Design review of the part built by this model. Coordinates are the model's own, in mm. A direction names the side the tool comes from. Round coordinates to 2 decimals unless told otherwise and drop trailing zeros. Order: outer loops, then holes, each group sorted by start corner. A loop starts at its lowest first (then second) coordinate and runs counter-clockwise, first axis right, second up. Notation, with made-up numbers: (58.5, 29.5) - (67.5, 29.5) arc R7 ccw to (67.5, 35.5) - close; hole circle Ø11 at (-36.75, 47.25). An arc over 180 degrees is marked (long way). Write item = value, one per line.
from build123d import *

# Parameters (mm, degrees)
SKETCH3_W           = 22.5
SKETCH3_H           = 23.5
BOSS_EXTRUDE1_DEPTH = 6.175
SKETCH4_W           = 12.35
SKETCH4_H           = 32
BOSS_EXTRUDE2_DEPTH = 2
BOSS_EXTRUDE3_DEPTH = 4.2
SKETCH6_R           = 2.5
CUT_EXTRUDE1_DEPTH  = 4.2
FILLET1_R           = 2
SKETCH7_R           = 2.5
BOSS_EXTRUDE4_DEPTH = 7.2
SKETCH8_R           = 1
CUT_EXTRUDE2_DEPTH  = 7


with BuildPart() as part:
    # Sketch3 → Boss-Extrude1 (new body, symmetric)
    with BuildSketch(Plane(origin=(0, -28.275548605, 0), x_dir=(0, 1, 0), z_dir=(1, 0, 0))):
        with Locations((24.609729517, 167.116706922)):
            Rectangle(SKETCH3_W, SKETCH3_H)
    extrude(amount=BOSS_EXTRUDE1_DEPTH, both=True)

    # Sketch4 → Boss-Extrude2 (add)
    with BuildSketch(Plane.XY.offset(174.666706922)):
        with Locations((0, -3.665819089)):
            Rectangle(SKETCH4_W, SKETCH4_H)
    extrude(amount=-BOSS_EXTRUDE2_DEPTH)

    # Sketch5 → Boss-Extrude3 (add)
    with BuildSketch(Plane.XY.offset(178.866706922)):
        with BuildLine():
            ThreePointArc((2.210095356, -3.993944089), (0, 7.584180911), (-2.210095356, -3.993944089))
            ThreePointArc((-2.210095356, -3.993944089), (0, -6.665819089), (2.210095356, -3.993944089))
        make_face()
    extrude(amount=BOSS_EXTRUDE3_DEPTH)

    # Sketch6 → Cut-Extrude1 (cut)
    with BuildSketch(Plane.XY.offset(183.066706922)):
        with Locations((0, 1.584180911)):
            Circle(SKETCH6_R)
    extrude(amount=-CUT_EXTRUDE1_DEPTH, mode=Mode.SUBTRACT)

    # Fillet1
    fillet1_edges = [part.edges().sort_by_distance(p)[0] for p in [
        (-6.175, -19.665819089, 173.666706922),
        (6.175, 12.334180911, 173.666706922),
        (-6.175, 12.334180911, 173.666706922),
        (6.175, -19.665819089, 173.666706922),
    ]]
    fillet(fillet1_edges, radius=FILLET1_R)

    # Sketch7 → Boss-Extrude4 (add)
    with BuildSketch(Plane.XY.offset(178.866706922)):
        with Locations((0, 1.584180911)):
            Circle(SKETCH7_R)
    extrude(amount=BOSS_EXTRUDE4_DEPTH)

    # Sketch8 → Cut-Extrude2 (cut)
    with BuildSketch(Plane.XY.offset(186.066706922)):
        with Locations((0, 1.584180911)):
            Circle(SKETCH8_R)
    extrude(amount=-CUT_EXTRUDE2_DEPTH, mode=Mode.SUBTRACT)


solid = part.part
1) We need section B-B on z = 158. Write out the cut boundary in (x, y) (3 decimals).
Findings:
outline = (-6.175, -14.916) - (6.175, -14.916) - (6.175, 7.584) - (-6.175, 7.584) - close
2) We need section A-A on y = -6. Write out the cut boundary in (x, z) (3 decimals), and give its area (3 significant figures).
Findings:
outline = (-6.175, 155.367) - (6.175, 155.367) - (6.175, 178.867) - (1.598, 178.867) - (1.598, 183.067) - (-1.598, 183.067) - (-1.598, 178.867) - (-6.175, 178.867) - close
area = 304 mm^2
3) For faces 1 (the flat face through (0, 7.584, 177)), 2 (the flat face through (0, -14.916, 177)), 3 (the flat face through (0, 7.584, 164)), 4 (the cylindrical face through (0.23, 7.58, 180.94)), list the 3-axis set-ups (+Z, -Z, +X, -X, +Y, -Y) from which the entire face can be reached by the end or side of a thin tool; tool diameter is ignored.
Findings:
face_1 = +Z, +X, -X, +Y
face_2 = +Z, +X, -X, -Y
face_3 = -Z, +X, -X, +Y
face_4 = +Z
4) The part is to be moulded in two halves that separate along X. For faces 5 (the flat face through (0, 10, 174.667)), 6 (the cylindrical face through (-0.13, 2.576, 182.616)), 7 (the cylindrical face through (-5.605, -19.064, 173.653)), say which applies: released by +X, released by -X, zero draft, split by the parting line, or undercut.
Findings:
face_5 = zero draft
face_6 = undercut
face_7 = released by -X
5) We need section C-C on x = -3. Write out the cut boundary in (y, z).
Findings:
outline = (-19.67, 172.67) - (-14.92, 172.67) - (-14.92, 155.37) - (7.58, 155.37) - (7.58, 172.67) - (12.33, 172.67) - (12.33, 174.67) - (7.58, 174.67) - (7.58, 178.87) - (6.78, 178.87) - (6.78, 183.07) - (-3.61, 183.07) - (-3.61, 178.87) - (-14.92, 178.87) - (-14.92, 174.67) - (-19.67, 174.67) - close
6) We need section D-D on z = 182. Write out the cut boundary in (x, y).
Findings:
outline = (-2.21, -3.99) arc R2.25 ccw (long way) to (2.21, -3.99) arc R6 ccw (long way) to start; hole circle Ø2 at (0, 1.58)
7) To check wall thickness, follow L1, parallel to Y at x = 0, z = 182.25; L2, parallel to Y at x = 0, z = 184.5; L3, parallel to Z at x = 4, y = -14. State the ranges of each line that lie inside material, in increasing order. Write a range as from..to.
Findings:
L1 = -6.67..0.58, 2.58..7.58
L2 = -0.92..0.58, 2.58..4.08
L3 = 155.37..178.87
8) Clearance check with flat-ended pins moving along their axes: pin 1 Ø1.5 at (x, z) = (-1, 162.5) entering from +Y; pin 2 Ø1.4 at (x, y) = (1, -18) entering from +Z; pin 3 Ø1.4 at (x, y) = (1, 10) entering from -Z. State where each tip first meets the part, or that it passes through.
Findings:
pin_1 = 7.58
pin_2 = 174.67
pin_3 = 172.67
